from build123d import *

# Parameters (mm, degrees)
F0_R     = 30
F1_DEPTH = 740
F2_W     = 100
F2_H     = 100
F2_R     = 30
F3_DEPTH = 5
F5_D     = 8.8


with BuildPart() as f1:
    # F0 (on Top) → F1 (new body)
    with BuildSketch(Plane.XY):
        Circle(F0_R)
    extrude(amount=F1_DEPTH)

    # F2 (on face) → F3 (join)
    with BuildSketch(Plane.XY.offset(740)):
        Rectangle(F2_W, F2_H)
        Circle(F2_R, mode=Mode.SUBTRACT)
        Circle(F2_R)
    extrude(amount=F3_DEPTH)

    # F5 (through all)
    with Locations(Plane.XY.offset(745)):
        with Locations((-40, 40), (40, 40), (40, -40), (-40, -40)):
            Hole(F5_D / 2)


solid = f1.part
Read the model definition and answer for the solid it produces. Units are mm, in the model's axes. A direction names the side the tool comes from. Coordinates: 2 decimals unless noted, no trailing zeros. Write each loop counter-clockwise with the first axis right and the second up, starting at its lowest first coordinate (ties: lowest second). Pieces come first, ordered by that corner, then holes. Notation, with made-up numbers: (-12.75, 34) -> (4.25, 34) arc R15 ccw to (4.25, 53) -> close; hole circle Ø11 at (6.25, 75.25). An arc over 180 degrees is marked (long way). Return JSON: item names as keys, results as strings.
(1) Which of the six approach directions +Z, -Z, +X, -X, +Y, -Y give full straight-line access (tool end or side, diameter ignored) to faces 1 (the flat face through (-1, 1, 745)), 2 (the cylindrical face through (-29.97, 1.32, 364.82))?
Answers below:
{"face 1": "+Z, +X, -X, +Y, -Y", "face 2": "-Z"}
(2) The part is cut by section B-B on x = -2. Give the vertices of the cut face in (y, z), then the cut area to 3 significant figures.
Answers below:
{"outline": "(-50, 740) -> (-29.93, 740) -> (-29.93, 0) -> (29.93, 0) -> (29.93, 740) -> (50, 740) -> (50, 745) -> (-50, 745) -> close", "area": "44,800 mm^2"}
(3) Each of these flat-tipped pins is pushed along its axis until it touches: P1, Ø1, axis at y = 19, z = 502.5, coming from the -X side; P2, Ø14, axis at x = 40, y = -40, coming from the -Z side; P3, Ø1, axis at x = 1.5, z = 416, coming from the -Y side; P4, Ø5, axis at x = -33, z = 160.5, coming from the +Y side. Where does it stop, or does it pass through?
Answers below:
{"P1": "x = -23.62", "P2": "z = 740", "P3": "y = -29.98", "P4": "through"}
(4) The part is cut by section C-C on z = 153.5. Give the vertices of the cut face in (x, y).
Answers below:
{"outline": "circle Ø60 at (0, 0)"}
(5) Consider line 1 along Y through (x, z) = (40, 742.9); line 2 along Z through (x, y) = (21.5, 38.5); line 3 along X through (y, z) = (3, 285.5). Determine where each line is inside the solid, lowest interval first. Write a range as from..to.
Answers below:
{"line 1": "-50..-44.4, -35.6..35.6, 44.4..50", "line 2": "740..745", "line 3": "-29.85..29.85"}
(6) The part is cut by section A-A on y = 0. Give the vertices of the cut face in (x, z).
Answers below:
{"outline": "(-50, 740) -> (-30, 740) -> (-30, 0) -> (30, 0) -> (30, 740) -> (50, 740) -> (50, 745) -> (-50, 745) -> close"}
